Model file for the job. Use its own axes, mm. Round coordinates to 2 decimals unless told otherwise and drop trailing zeros. Loops run counter-clockwise (first coordinate to the right, second up) from the corner with the lowest first, then second, coordinate; pieces in that order, holes last. Notation, with made-up numbers: (48, -40) - (96, -40) arc R21 ccw to (96, -13) - close; hole circle Ø6 at (52, 88). An arc over 180 degrees is marked (long way). Answer as a JSON object with one key per item and string values.
from build123d import *

# Parameters (mm, degrees)
BOSS_EXTRUDE1_DEPTH = 215.9
SKETCH2_W           = 65
SKETCH2_H           = 4.6
CUT_EXTRUDE1_DEPTH  = 229.165913841


with BuildPart() as part:
    # Sketch1 → Boss-Extrude1 (new body)
    with BuildSketch(Plane.XY):
        Polygon((187.42097357, 132.785097993), (137.579115796, 174.124053731), (138.600551034, 175.35558532), (188.63152184, 133.859778782), (193.220657018, 125.592655419), (194.701118326, 119.670240299), align=None)
    extrude(amount=-BOSS_EXTRUDE1_DEPTH)

    # Sketch2 → Cut-Extrude1 (cut, through all)
    with BuildSketch(Plane(origin=(142.652779273, 171.994657551, 0), x_dir=(0.7697072431709691, -0.6383970236538912, 0), z_dir=(0.6383970236538911, 0.769707243170969, 0))):
        with Locations((27.235364289, 2.3)):
            Rectangle(SKETCH2_W, SKETCH2_H)
        with Locations((27.235364289, 213.6)):
            Rectangle(SKETCH2_W, SKETCH2_H)
    extrude(amount=-CUT_EXTRUDE1_DEPTH, mode=Mode.SUBTRACT)


solid = part.part
1) Probe probe 1 along X at (y, z) = (170, -27); probe 2 along Z at (x, y) = (148.5, 167); probe 3 along X at (y, z) = (158.5, -70). List the from-to ranges inside material, lowest first.
Values follow:
{"probe 1": "142.55 to 145.06", "probe 2": "-211.3 to -4.6", "probe 3": "156.42 to 158.92"}
2) Slice it at C-C on x = 150.5. List the corners of the cut face in (y, z), then the cut area to 3 significant figures.
Values follow:
{"outline": "(163.41, -211.3) - (165.49, -211.3) - (165.49, -4.6) - (163.41, -4.6) - close", "area": "430 mm²"}
3) Slice it at A-A on z = -100. List the corners of the cut face in (x, y), then the cut area to 3 significant figures.
Values follow:
{"outline": "(137.58, 174.12) - (187.42, 132.79) - (194.7, 119.67) - (193.22, 125.59) - (188.63, 133.86) - (138.6, 175.36) - close", "area": "123 mm²"}
4) Drop flat-ended pins along their axis: P1, Ø10, axis at x = 163.5, z = -130, coming from the +Y side; P2, Ø1.5, axis at y = 143, z = -110, coming from the +X side; P3, Ø10, axis at x = 176.5, z = -103.5, coming from the +Y side. Give the stop position or say it passes through.
Values follow:
{"P1": "y = 158.85", "P2": "x = 178.52", "P3": "y = 148.07"}
5) Slice it at B-B on y = 130.5. List the corners of the cut face in (x, z), then the cut area to 3 significant figures.
Values follow:
{"outline": "(188.69, -215.9) - (190.5, -215.9) - (190.5, 0) - (188.69, 0) - close", "area": "390 mm²"}
